Could you check a few things on this drawing? It's one solid part, dimensions in mm from its lowest x, y, z. A direction names the side the tool comes from. Coordinates: 2 decimals unless noted, no trailing zeros. Order: outer loops, then holes, each group sorted by start corner. A loop starts at its lowest first (then second) coordinate and runs counter-clockwise, first axis right, second up. Notation, with made-up numbers: (3.25, 18.5) -> (33.25, 18.5) arc R36 ccw to (33.25, 57.5) -> close; hole circle Ø10 at (62, -12). An arc over 180 degrees is marked (long way). Use a Markdown table: item, result. Add a question column.
1. Suppose I cut it at C-C, the plane z = 46.5. List the corners of the cut face in (x, y) for me.
2. For the marked faces 1, 2 and 3, which set-ups out of +Z, -Z, +X, -X, +Y, -Y let a thin tool reach every point of the face, with its end or its side?
3. If I drill on line 1 along X through (y, z) = (1.5, 29.21); line 2 along Z through (x, y) = (14.5, 6.25); line 3 along X through (y, z) = (11.5, 24), over which ranges is the centre line in solid material (lowest first)? Write a range as from..to.
4. Suppose I cut it at A-A, the plane z = 29.21. List the corners of the cut face in (x, y) for me, then the cut area to 3 significant figures.
5. Suppose I cut it at D-D, the plane y = 18. List the corners of the cut face in (x, z) for me.
6. For pin 1 Ø5 at (x, y) = (38, 18) entering from +Z; pin 2 Ø8 at (y, z) = (14.5, 36) entering from -X; pin 3 Ø10 at (y, z) = (9, 7) entering from +X, each with a flat end and sliding along its axis, tell me the tip position at first contact or that it passes through.
7. Suppose I cut it at B-B, the plane x = 20.5. List the corners of the cut face in (y, z) for me, then the cut area to 3 significant figures.
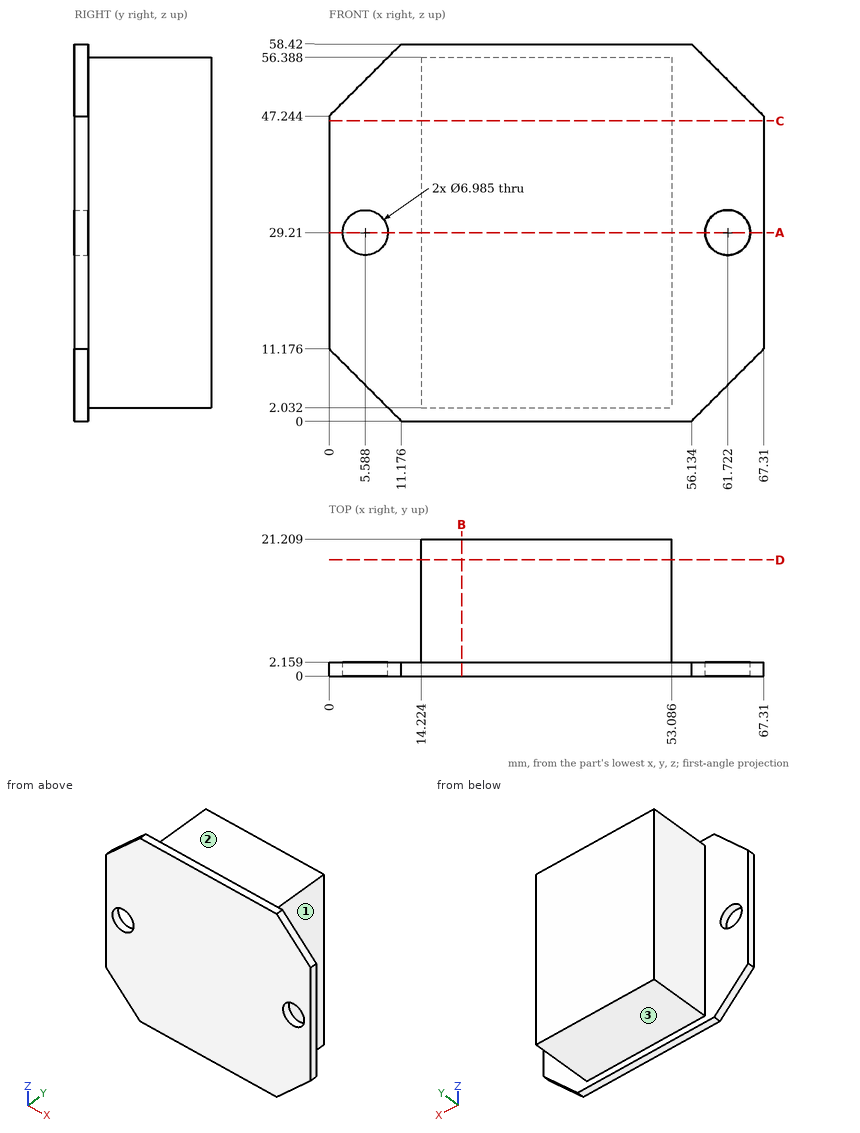
Worked out:
| question | item | result |
|---|---|---|
| 1 | outline | (0, 0) -> (67.31, 0) -> (67.31, 2.16) -> (53.09, 2.16) -> (53.09, 21.21) -> (14.22, 21.21) -> (14.22, 2.16) -> (0, 2.16) -> close |
| 2 | face 1 | +Z, -Z, +X, +Y |
| 2 | face 2 | +Z, +X, -X, +Y |
| 2 | face 3 | -Z, +X, -X, +Y |
| 3 | line 1 | x = 0..2.1, 9.08..58.23, 65.21..67.31 |
| 3 | line 2 | z = 2.03..56.39 |
| 3 | line 3 | x = 14.22..53.09 |
| 4 | outline | (0, 0) -> (2.1, 0) -> (2.1, 2.16) -> (0, 2.16) -> close; (9.08, 0) -> (58.23, 0) -> (58.23, 2.16) -> (53.09, 2.16) -> (53.09, 21.21) -> (14.22, 21.21) -> (14.22, 2.16) -> (9.08, 2.16) -> close; (65.21, 0) -> (67.31, 0) -> (67.31, 2.16) -> (65.21, 2.16) -> close |
| 4 | area | 855 mm² |
| 5 | outline | (14.22, 2.03) -> (53.09, 2.03) -> (53.09, 56.39) -> (14.22, 56.39) -> close |
| 6 | pin 1 | stops at z = 56.39 |
| 6 | pin 2 | stops at x = 14.22 |
| 6 | pin 3 | stops at x = 53.09 |
| 7 | outline | (0, 0) -> (2.16, 0) -> (2.16, 2.03) -> (21.21, 2.03) -> (21.21, 56.39) -> (2.16, 56.39) -> (2.16, 58.42) -> (0, 58.42) -> close |
| 7 | area | 1,160 mm² |
